The drawing under review shows one solid part. Ordinate dimensions are in mm from its lowest x, y, z. A direction names the side the tool comes from. Give positions to 0.01 mm unless a question says otherwise; leave off trailing zeros. Write each loop counter-clockwise with the first axis right and the second up, starting at its lowest first coordinate (ties: lowest second). Pieces come first, ordered by that corner, then holes. Notation, with made-up numbers: (-13.5, 34) -> (38.5, 34) arc R25 ccw to (38.5, 62) -> close; hole circle Ø6 at (5.25, 77.25). An arc over 180 degrees is marked (long way). Answer as a JSON object with one key per item and string values.
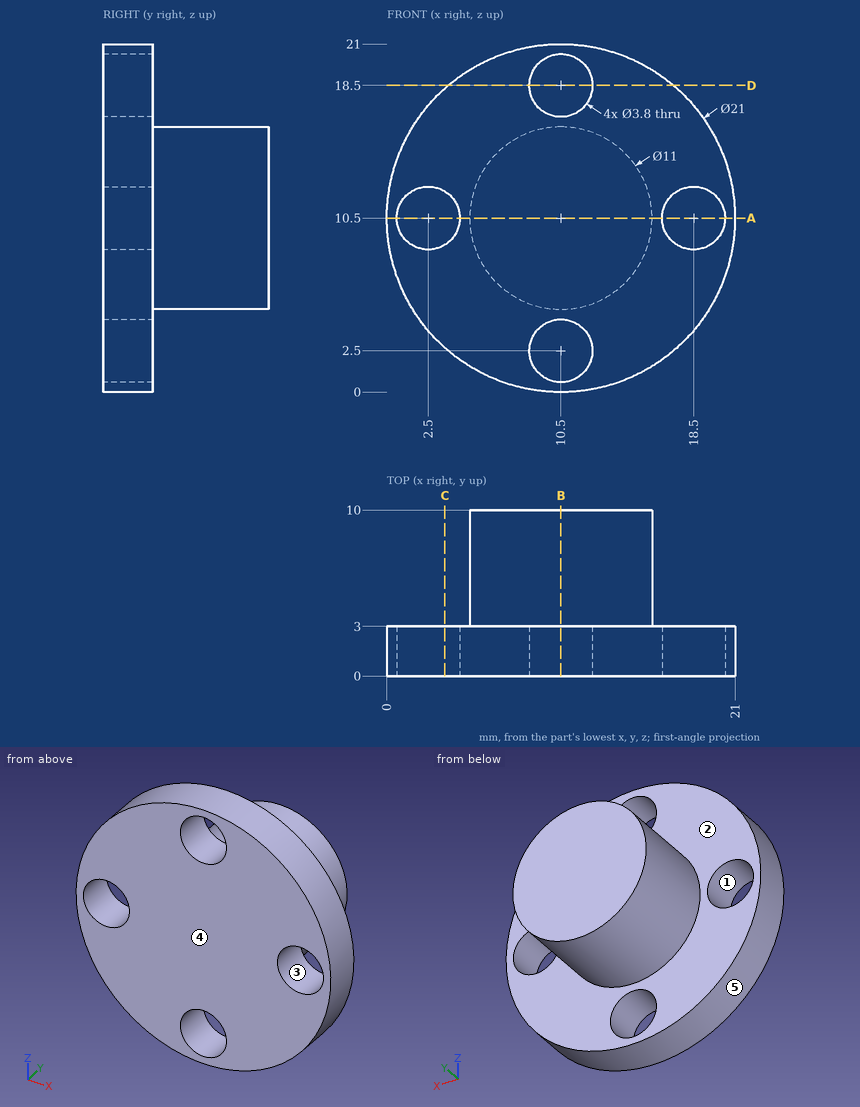
(1) The part is to be moulded in two halves that separate along X. For the marked faces 3, 4 and 5, say which applies: +X half, -X half, draft (parallel to the pull), parting line (faces both ways), or undercut.
Here are the results:
{"face 3": "undercut", "face 4": "draft", "face 5": "parting line"}
(2) We need section B-B, the plane x = 10.5. State the section outline as (y, z) points, then the cut area to 3 significant figures.
Here are the results:
{"outline": "(0, 0) -> (3, 0) -> (3, 0.6) -> (0, 0.6) -> close; (0, 4.4) -> (3, 4.4) -> (3, 5) -> (10, 5) -> (10, 16) -> (3, 16) -> (3, 16.6) -> (0, 16.6) -> close; (0, 20.4) -> (3, 20.4) -> (3, 21) -> (0, 21) -> close", "area": "117 mm²"}
(3) For line 1 along X through (y, z) = (1.4, 10.5); line 2 along X through (y, z) = (2, 17.25); line 3 along Y through (x, z) = (7.25, 3.75), list the stretches that pass through material, from the lowest coordinate up.
Here are the results:
{"line 1": "x = 0 to 0.6, 4.4 to 16.6, 20.4 to 21", "line 2": "x = 2.46 to 9.07, 11.93 to 18.54", "line 3": "y = 0 to 3"}
(4) We need section C-C, the plane x = 3.5. State the section outline as (y, z) points.
Here are the results:
{"outline": "(0, 2.67) -> (3, 2.67) -> (3, 8.88) -> (0, 8.88) -> close; (0, 12.12) -> (3, 12.12) -> (3, 18.33) -> (0, 18.33) -> close"}
(5) For the marked faces 1 and 2, list the 3-axis set-ups (+Z, -Z, +X, -X, +Y, -Y) from which the entire face can be reached by the end or side of a thin tool; tool diameter is ignored.
Here are the results:
{"face 1": "+Y, -Y", "face 2": "+Y"}
(6) Clearance check with flat-ended pins moving along their axes: pin 1 (2 mm diameter, centred on y = 4.5, z = 6.5, fed in from +X); pin 2 (5 mm diameter, centred on x = 12.5, z = 2.5, fed in from -Y); pin 3 (5 mm diameter, centred on x = 16, y = 8, fed in from +Z); pin 4 (1 mm diameter, centred on x = 5.5, y = 7.5, fed in from +Z). State where each tip first meets the part, or that it passes through.
Here are the results:
{"pin 1": "stops at x = 15.11", "pin 2": "stops at y = 0", "pin 3": "stops at z = 15.11", "pin 4": "stops at z = 13.66"}
(7) We need section D-D, the plane z = 18.5. State the section outline as (x, y) points, then the cut area to 3 significant figures.
Here are the results:
{"outline": "(3.7, 0) -> (8.6, 0) -> (8.6, 3) -> (3.7, 3) -> close; (12.4, 0) -> (17.3, 0) -> (17.3, 3) -> (12.4, 3) -> close", "area": "29.4 mm²"}
(8) We need section A-A, the plane z = 10.5. State the section outline as (x, y) points, then the cut area to 3 significant figures.
Here are the results:
{"outline": "(0, 0) -> (0.6, 0) -> (0.6, 3) -> (0, 3) -> close; (4.4, 0) -> (16.6, 0) -> (16.6, 3) -> (16, 3) -> (16, 10) -> (5, 10) -> (5, 3) -> (4.4, 3) -> close; (20.4, 0) -> (21, 0) -> (21, 3) -> (20.4, 3) -> close", "area": "117 mm²"}
